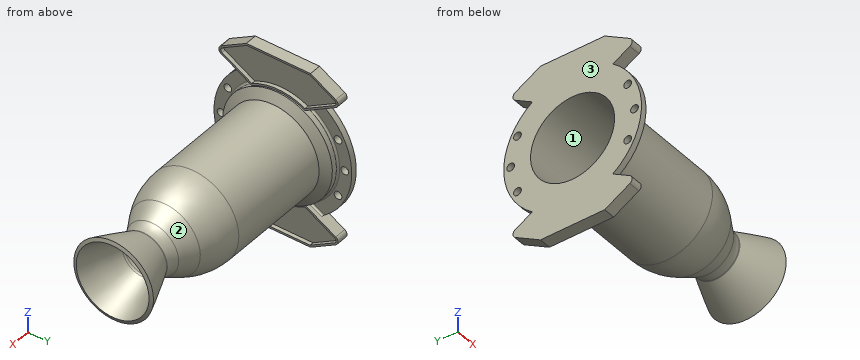
```python
from build123d import *
from build123d.topology import SkipClean

# Parameters (mm, degrees)
BOSS_EXTRUDE1_DEPTH = 16.256
CUT_EXTRUDE1_DEPTH  = 5.334
BOSS_EXTRUDE2_START = -8.128
BOSS_EXTRUDE2_DEPTH = 8.128
FILLET2_R           = 2.54
SKETCH9_R           = 5.276996688
CUT_EXTRUDE2_DEPTH  = 344.8417333


with BuildPart() as part:
    # Sketch3 → Revolve1 (revolve)
    with BuildSketch(Plane.XY, mode=Mode.PRIVATE) as revolve1_sk:
        with BuildLine():
            Line((0, 62.50116278), (144.934662069, 62.50116278))
            ThreePointArc((144.934662069, 62.50116278), (171.563195097, 58.995430145), (196.377031865, 48.717179445))
            Line((196.377031865, 48.717179445), (218.627148666, 35.871044168))
            ThreePointArc((218.627148666, 35.871044168), (225.918357505, 32.850926621), (233.742787922, 31.820817416))
            ThreePointArc((233.742787922, 31.820817416), (234.25849688, 31.874994553), (234.751688107, 32.035161047))
            add(Edge.make_bspline(
                [(234.751688107, 32.035161047), (237.01563786, 33.042605222), (241.558012865, 35.047750332), (250.598858454, 38.973761134), (261.865302755, 43.744407277), (273.069848062, 48.325693823), (282.005645487, 51.880791718), (286.451986012, 53.616927894), (288.682041358, 54.479389474)],
                knots=[0, 0, 0, 0, 0.049644807, 0.099289614, 0.198579228, 0.297868842, 0.347513649, 0.397158456, 0.397158456, 0.397158456, 0.397158456], degree=3))
            Line((288.682041358, 54.479389474), (290.485579361, 49.816005438))
            add(Edge.make_bspline(
                [(236.784472704, 27.467044719), (254.870236719, 35.51510214), (272.770570963, 42.964823847), (290.485579361, 49.816005438)],
                knots=[0, 0, 0, 0, 0.397158456, 0.397158456, 0.397158456, 0.397158456], degree=3))
            ThreePointArc((236.784472704, 27.467044719), (235.297572794, 26.98416423), (233.742784709, 26.820827416))
            ThreePointArc((233.742784709, 26.820827416), (224.624261333, 28.021308096), (216.127150111, 31.540927862))
            Line((216.127150111, 31.540927862), (193.87703331, 44.387063139))
            ThreePointArc((193.87703331, 44.387063139), (170.269100478, 54.165811204), (144.934662069, 57.50117278))
            Line((144.934662069, 57.50117278), (0, 57.50117278))
            Line((0, 57.50117278), (0, 62.50116278))
        make_face()
    revolve(revolve1_sk.sketch.rotate(Axis((0, 0, 0), (1, 0, 0)), 90), axis=Axis((0, 0, 0), (1, 0, 0)))

    # Sketch4 → Revolve5 (revolve)
    with BuildSketch(Plane.XY, mode=Mode.PRIVATE) as revolve5_sk:
        Polygon((-25.4, 57.50117278), (-25.4, 75.20116278), (-7.332348419, 75.20116278), (0, 62.50116278), (0, 57.50117278), align=None)
    revolve(revolve5_sk.sketch.rotate(Axis((0, 0, 0), (1, 0, 0)), 90), axis=Axis((0, 0, 0), (1, 0, 0)))

    # Sketch6 → Boss-Extrude1 (add)
    with SkipClean():  # the faces are left unmerged after this step: merging them gives an invalid solid
        with BuildSketch(Plane.ZY.offset(25.4)):
            with BuildLine():
                Line((54.820128271, 17.35333995), (90.051671459, 78.37616278))
                ThreePointArc((90.051671459, 78.37616278), (95.550932773, 81.55116278), (101.050194087, 78.37616278))
                Line((101.050194087, 78.37616278), (120.950932773, 43.907072268))
                Line((120.950932773, 43.907072268), (120.950932773, -43.907072268))
                Line((120.950932773, -43.907072268), (101.050194087, -78.37616278))
                ThreePointArc((101.050194087, -78.37616278), (95.550932773, -81.55116278), (90.051671459, -78.37616278))
                Line((90.051671459, -78.37616278), (54.820128271, -17.35333995))
                ThreePointArc((54.820128271, -17.35333995), (57.50117278, 0), (54.820128271, 17.35333995))
            make_face()
            with BuildLine():
                Line((-54.820128271, -17.35333995), (-90.051671459, -78.37616278))
                ThreePointArc((-90.051671459, -78.37616278), (-95.550932773, -81.55116278), (-101.050194087, -78.37616278))
                Line((-101.050194087, -78.37616278), (-120.950932773, -43.907072268))
                Line((-120.950932773, -43.907072268), (-120.950932773, 43.907072268))
                Line((-120.950932773, 43.907072268), (-101.050194087, 78.37616278))
                ThreePointArc((-101.050194087, 78.37616278), (-95.550932773, 81.55116278), (-90.051671459, 78.37616278))
                Line((-90.051671459, 78.37616278), (-54.820128271, 17.35333995))
                ThreePointArc((-54.820128271, 17.35333995), (-57.50117278, 0), (-54.820128271, -17.35333995))
            make_face()
        extrude(amount=-BOSS_EXTRUDE1_DEPTH)

    # Sketch7 → Cut-Extrude1 (cut)
    with SkipClean():  # the faces are left unmerged after this step: merging them gives an invalid solid
        with BuildSketch(Plane(origin=(-9.144, 0, 0), x_dir=(0, 0, -1), z_dir=(1, 0, 0))):
            with BuildLine():
                Line((-68.720104511, 36.34880502), (-92.251375985, 77.10616278))
                ThreePointArc((-92.251375985, 77.10616278), (-95.550932773, 79.01116278), (-98.850489562, 77.10616278))
                Line((-98.850489562, 77.10616278), (-118.410932773, 43.226481319))
                Line((-118.410932773, 43.226481319), (-118.410932773, -43.226481319))
                Line((-118.410932773, -43.226481319), (-98.850489562, -77.10616278))
                ThreePointArc((-98.850489562, -77.10616278), (-95.550932773, -79.01116278), (-92.251375985, -77.10616278))
                Line((-92.251375985, -77.10616278), (-68.720104511, -36.34880502))
                ThreePointArc((-68.720104511, -36.34880502), (-77.74116278, 0), (-68.720104511, 36.34880502))
            make_face()
            with BuildLine():
                Line((92.251375985, -77.10616278), (68.720104511, -36.34880502))
                ThreePointArc((68.720104511, -36.34880502), (77.74116278, 0), (68.720104511, 36.34880502))
                Line((68.720104511, 36.34880502), (92.251375985, 77.10616278))
                ThreePointArc((92.251375985, 77.10616278), (95.550932773, 79.01116278), (98.850489562, 77.10616278))
                Line((98.850489562, 77.10616278), (118.410932773, 43.226481319))
                Line((118.410932773, 43.226481319), (118.410932773, -43.226481319))
                Line((118.410932773, -43.226481319), (98.850489562, -77.10616278))
                ThreePointArc((98.850489562, -77.10616278), (95.550932773, -79.01116278), (92.251375985, -77.10616278))
            make_face()
        extrude(amount=-CUT_EXTRUDE1_DEPTH, mode=Mode.SUBTRACT)

    # Sketch8 → Boss-Extrude2 (add)
    with SkipClean():  # the faces are left unmerged after this step: merging them gives an invalid solid
        with BuildSketch(Plane.ZY.offset(25.4).offset(BOSS_EXTRUDE2_START)):
            with BuildLine():
                Line((-65.810567847, -36.389339691), (-76.548297649, -54.987633268))
                ThreePointArc((-76.548297649, -54.987633268), (0, -94.25116278), (76.548297649, -54.987633268))
                Line((76.548297649, -54.987633268), (65.810567847, -36.389339691))
                ThreePointArc((65.810567847, -36.389339691), (0, -75.20116278), (-65.810567847, -36.389339691))
            make_face()
            with BuildLine():
                Line((76.548297649, 54.987633268), (65.810567847, 36.389339691))
                ThreePointArc((65.810567847, 36.389339691), (0, 75.20116278), (-65.810567847, 36.389339691))
                Line((-65.810567847, 36.389339691), (-76.548297649, 54.987633268))
                ThreePointArc((-76.548297649, 54.987633268), (0, 94.25116278), (76.548297649, 54.987633268))
            make_face()
        extrude(amount=BOSS_EXTRUDE2_DEPTH)

    # Fillet2
    fillet2_edges = [part.edges().sort_by_distance(p)[0] for p in [
        (-17.272, 75.20116278, 0),
        (-17.272, 45.68848648, -71.179432748),
        (-17.272, 45.68848648, 71.179432748),
        (-17.272, -75.20116278, 0),
        (-17.272, -45.68848648, 71.179432748),
        (-17.272, -45.68848648, -71.179432748),
    ]]
    fillet(fillet2_edges, radius=FILLET2_R)

    # Sketch9 → Cut-Extrude2 (cut, through all)
    with SkipClean():  # the faces are left unmerged after this step: merging them gives an invalid solid
        with BuildSketch(Plane(origin=(-17.272, 0, 0), x_dir=(0, 0, -1), z_dir=(1, 0, 0))):
            with Locations((-38.668190551, 75.387622983)):
                Circle(SKETCH9_R)
            with Locations((0.000121249, 84.72616278)):
                Circle(SKETCH9_R)
            with Locations((38.66840632, 75.387512308)):
                Circle(SKETCH9_R)
            with Locations(Location((38.66840632, -75.387512308, 0), (0, 0, 180))):
                Circle(SKETCH9_R)
            with Locations(Location((0.000121249, -84.72616278, 0), (0, 0, 180))):
                Circle(SKETCH9_R)
            with Locations(Location((-38.668190551, -75.387622983, 0), (0, 0, 180))):
                Circle(SKETCH9_R)
        extrude(amount=-CUT_EXTRUDE2_DEPTH, mode=Mode.SUBTRACT)


solid = part.part
```
Geometry: final body of the model. Coordinates: model frame, mm. Face numbers are marked on the shaded views. Round coordinates to 2 decimals unless told otherwise and drop trailing zeros. Write item = value, one per line. Start each with the question number.
Q1. Ray query, line 1 (Y direction, x = 183, z = -12); line 2 (Z direction, x = 169.5, y = -28). Return the intervals inside material, ascending. Write a range as from..to.
Q2. Pin query (flat end, axial travel): pin 1 (10 mm diameter, centred on x = 141.5, z = -31, fed in from +Y); pin 2 (2 mm diameter, centred on x = 246, y = -34, fed in from -Z); pin 3 (6.5 mm diameter, centred on y = -75.39, z = -38.67, fed in from -X); pin 4 (3 mm diameter, centred on x = 203, y = 9.5, fed in from -Z). Return the tip coordinate at first contact, or that it passes through.
Q3. Pull-direction query (Y, two-part tool) for the marked faces 1, 2 and 3; classes: +Y half, -Y half, draft (parallel to the pull), parting line (faces both ways), or undercut.
Outcome:
q1.line_1 = -53.88..-48.33, 48.33..53.88
q1.line_2 = -52.53..-46.6, 46.6..52.53
q2.pin_1 = 56.84
q2.pin_2 = -16.9
q2.pin_3 = through
q2.pin_4 = -44.82
q3.face_1 = undercut
q3.face_2 = parting line
q3.face_3 = draft
